Autodesk Fusion 360 part; units mm, degrees
sketch "Sketch1" plane through (0, 0, 0) normal (0, 0, 1) x (1, 0, 0)
  line L0 (20, -11) -> (-20, -11)
  line L1 (-20, -11) -> (-20, 11)
  line L2 (-20, 11) -> (20, 11)
  line L3 (20, 11) -> (20, -11)
  line L4 (20, -11) -> (-20, 11) construction
  line L5 (-20, -11) -> (20, 11) construction
  line L6 (20, 11) -> (35, 11)
  line L7 (35, 11) -> (35, -11)
  line L8 (35, -11) -> (20, -11)
  line L9 (20, -11) -> (20, 11)
  line L10 (-20, 11) -> (-35, 11)
  line L11 (-35, 11) -> (-35, -11)
  line L12 (-35, -11) -> (-20, -11)
  line L13 (-20, -11) -> (-20, 11)
  line L14 (-35, 0) -> (35, 0)
  circle A0 centre (27.5, 0) radius 2.65
  circle A1 centre (27.5, 0) radius 5.5 construction
  line L15 (27.5, 11) -> (27.5, -11) construction
  line L16 (-27.5, 11) -> (-27.5, -11) construction
  circle A2 centre (-27.5, 0) radius 2.65
  line L17 (-20, 3) -> (20, 3)
  line L18 (-20, -4) -> (20, -4) construction
  circle A3 centre (14, -4) radius 2.55
  circle A4 centre (-14, -4) radius 2.55
  line L19 (-35, 1.5) -> (35, 1.5) construction
  line L20 (-35, -1.5) -> (35, -1.5) construction
  circle A5 centre (-27.5, 1.5) radius 2.65
  circle A6 centre (-27.5, -1.5) radius 2.65
  circle A7 centre (27.5, -1.5) radius 2.65
  circle A8 centre (27.5, 1.5) radius 2.65
  line L21 (24.85, 1.5) -> (24.85, -1.5)
  line L22 (30.15, 1.5) -> (30.15, -1.5)
  line L23 (-30.15, 1.5) -> (-30.15, -1.5)
  line L24 (-24.85, 1.5) -> (-24.85, -1.5)
  dimension "d1" = 22
  dimension "d2" = 40
  dimension "d3" = 15
  dimension "d4" = 15
  dimension "d5" = 5.3
  dimension "d6" = 11
  dimension "d7" = 5.3
  dimension "d21" = 14
  dimension "d22" = 7
  dimension "d23" = 5.1
  dimension "d24" = 5.1
  dimension "d25" = 6
  dimension "d26" = 6
  dimension "d32" = 1.5
  dimension "d33" = 1.5
  dimension "d34" = 5.3
  dimension "d35" = 5.3
  dimension "d36" = 5.3
  dimension "d37" = 5.3
  dimension "d40" = 28
  dimension "d41" = 55
  dimension "d42" = 13.5
extrude "Extrude2" add sketch "Sketch1" along normal blind 43.5 contours L0 L1 L3 L9 L13 L14 | L1 L3 L9 L13 L14 L17 | A3 | A4
extrude "Extrude1" add sketch "Sketch1" along normal blind 5 contours L3 L7 L8 L9 L14 A7 L21 L22 | L1 L11 L12 L13 L14 A6 L23 L24 | L3 L6 L7 L9 L14 A8 L21 L22 | L1 L10 L11 L13 L14 A5 L23 L24 | L1 L2 L3 L9 L13 L17
extrude "Extrude4" cut sketch "Sketch1" against normal blind 10 from surface at 43.5 contours A3 | A4
fillet "Fillet3" radius 3 4 edges at (-35, -11, 2.5) (-35, 11, 2.5) (35, 11, 2.5) (35, -11, 2.5)
chamfer "Chamfer2" distance 1 angle 45 3 edges at (20, -4, 5) (0, 3, 5) (-20, -4, 5)
chamfer "Chamfer3" distance 1 angle 45 6 edges at (20, -11, 24.75) (20, 3, 24.75) (-20, 3, 24.75) (-20, -11, 24.75) (-20.5, 3.5, 5.5) (20.5, 3.5, 5.5)
chamfer "Chamfer1" [suppressed]
equation "d4 = d3"
equation "d7 = d5"
equation "d22 = ( d21 ) / 2"
equation "d24 = d23"
equation "d26 = d25"
equation "d33 = d32"
equation "d34 = d5"
equation "d35 = d5"
equation "d36 = d5"
equation "d37 = d5"
Part model, mm, in its own coordinate system. A direction names the side the tool comes from. Round coordinates to 2 decimals unless told otherwise and drop trailing zeros. Write each loop counter-clockwise with the first axis right and the second up, starting at its lowest first coordinate (ties: lowest second). Pieces come first, ordered by that corner, then holes. Notation, with made-up numbers: M 56,75 L 83,75 A18 ccw 83,98 Z; hole C 78,-16.75 d3. An arc over 180 degrees is marked long. Return JSON: item names as keys, results as strings. Group by question number.
(1) Drill centre lines: probe 1 along Y at (x, z) = (14, 41.25); probe 2 along X at (y, z) = (-1.25, 19.5); probe 3 along Y at (x, z) = (-2, 29). Where is each one in solid material? Low to high.
(2) Saw through at A-A on y = -0.5. Write the cut outline in (x, z).
(3) Saw through at D-D on z = 27. Write the cut outline in (x, y).
(4) Saw through at B-B on x = -27.5. Write the cut outline in (y, z), then the cut area to 3 significant figures.
(5) Two-plate mould, pull along X, no slides. Class faces 1 (the face through (14, -4, 33.5)), 2 (the face through (0, -11, 21)), 3 (the face through (35, 0, 2)): +X half, -X half, draft (parallel to the pull), parting line (faces both ways), or undercut.
(6) Saw through at C-C on z = 3.5. Write the cut outline in (x, y).
(7) Which spindle directions (+Z, -Z, +X, -X, +Y, -Y) get a long thin tool onto all of the face, cutting with end or side? Do faces 4 (the face through (0, 5, 5)), 5 (the face through (0, 3, 24)), 6 (the face through (-14, -4, 33.5)). Say none if no direction does.
(8) Pin check, flat tips, straight feed: pin 1 Ø12 at (x, z) = (-23, 33.5) entering from +Y; pin 2 Ø2.5 at (x, y) = (14.5, -4.5) entering from +Z; pin 3 Ø5 at (x, y) = (26.5, -6.5) entering from +Z. Stop position of each tip, or through.
Returned:
{
 "1": {"probe 1": "-11 to -6.55, -1.45 to 3", "probe 2": "-20 to 20", "probe 3": "-11 to 3"},
 "2": {"outline": "M -35,0 L -30.15,0 L -30.15,5 L -35,5 Z; M -24.85,0 L 24.85,0 L 24.85,5 L 21,5 L 20,6 L 20,43.5 L -20,43.5 L -20,6 L -21,5 L -24.85,5 Z; M 30.15,0 L 35,0 L 35,5 L 30.15,5 Z"},
 "3": {"outline": "M -20,-10 L -19,-11 L 19,-11 L 20,-10 L 20,2 L 19,3 L -19,3 L -20,2 Z"},
 "4": {"outline": "M -11,0 L -4.15,0 L -4.15,5 L -11,5 Z; M 4.15,0 L 11,0 L 11,5 L 4.15,5 Z", "area": "68.5 mm²"},
 "5": {"face 1": "undercut", "face 2": "draft", "face 3": "+X half"},
 "6": {"outline": "M -35,-8 A3 ccw -32,-11 L 32,-11 A3 ccw 35,-8 L 35,8 A3 ccw 32,11 L -32,11 A3 ccw -35,8 Z; hole M -30.15,-1.5 A2.65 ccw -24.85,-1.5 L -24.85,1.5 A2.65 ccw -30.15,1.5 Z; hole M 24.85,-1.5 A2.65 ccw 30.15,-1.5 L 30.15,1.5 A2.65 ccw 24.85,1.5 Z"},
 "7": {"face 4": "+Z, +Y", "face 5": "+Z, +X, -X, +Y", "face 6": "+Z"},
 "8": {"pin 1": "y = 3", "pin 2": "z = 33.5", "pin 3": "z = 5"}
}
